Work out the finished part from the listing and answer in its coordinate system (mm). Face numbers are marked on the shaded views. A direction names the side the tool comes from. Give positions to 0.01 mm unless a question says otherwise; leave off trailing zeros. Loops run counter-clockwise (first coordinate to the right, second up) from the corner with the lowest first, then second, coordinate; pieces in that order, holes last. Notation, with made-up numbers: (45.5, 80) - (79.5, 80) arc R23 cw to (79.5, 98) - close; hole circle Ø5 at (45.5, 5.25). An arc over 180 degrees is marked (long way). One line per question, with ' | ' between items.
from build123d import *

# Parameters (mm, degrees)
CUT_CENTER_DEPTH               = 53.414934066
CUT_CENTER_DEPTH_BACK          = 53.414934066
SKETCH_CENTER_CUT_R            = 12.5
CBORE_FOR_M6_SHCS1_D           = 6.6
CBORE_FOR_M6_SHCS1_CBORE_D     = 11
CBORE_FOR_M6_SHCS1_CBORE_DEPTH = 6
CIRPATTERN1_COUNT              = 6
SKETCH1_R                      = 14.25575
CUT_EXTRUDE1_DEPTH             = 3.9624
CUT_EXTRUDE2_DEPTH             = 6
CIRPATTERN2_COUNT              = 6


with BuildPart() as part:
    # Sketch Spindle Skeleton → Main Revolve (revolve)
    with BuildSketch(Plane(origin=(0, 0, 0), x_dir=(0, 0, -1), z_dir=(1, 0, 0)), mode=Mode.PRIVATE) as main_revolve_sk:
        Polygon((-26.320999936, -22.6187), (-26.320999936, -36.5125), (-17.320999902, -36.5125), (-17.320999902, -9.525), (-26.320999936, -9.525), (-26.320999936, -12.5), (-28.321, -12.5), (-28.321, -22.6187), align=None)
        Polygon((-26.320999936, 36.5125), (-26.320999936, 22.6187), (-28.321, 22.6187), (-28.321, 12.5), (-26.320999936, 12.5), (-26.320999936, 9.525), (-17.320999902, 9.525), (-17.320999902, 36.5125), align=None)
    revolve(main_revolve_sk.sketch.rotate(Axis((0, 0, 1000), (0, 0, -1)), 270), axis=Axis((0, 0, 1000), (0, 0, -1)))

    # Sketch Center Cut → Cut Center (cut, two sides: drawn at the far end of the back side and taken through both)
    with BuildSketch(Plane.XY.offset(26.320999936).offset(-CUT_CENTER_DEPTH_BACK)):
        Circle(SKETCH_CENTER_CUT_R)
    extrude(amount=CUT_CENTER_DEPTH + CUT_CENTER_DEPTH_BACK, mode=Mode.SUBTRACT)

    # CBORE for M6 SHCS1 (through all)
    with Locations(Plane(origin=(0, 0, 17.320999902), x_dir=(-1, 0, 0), z_dir=(0, 0, -1))):
        with Locations((0, 30.565600032)):
            cbore_for_m6_shcs1 = CounterBoreHole(CBORE_FOR_M6_SHCS1_D / 2, CBORE_FOR_M6_SHCS1_CBORE_D / 2, CBORE_FOR_M6_SHCS1_CBORE_DEPTH)

    # CirPattern1: CBORE for M6 SHCS1 ×6 about axis
    cirpattern1_axis = Axis((0, 0, 0), (0, 0, 1))
    for i in range(1, CIRPATTERN1_COUNT):
        add(cbore_for_m6_shcs1.rotate(cirpattern1_axis, i * 360 / CIRPATTERN1_COUNT), mode=Mode.SUBTRACT)

    # Sketch1 → Cut-Extrude1 (cut)
    with BuildSketch(Plane(origin=(0, 0, 17.320999902), x_dir=(-1, 0, 0), z_dir=(0, 0, -1))):
        Circle(SKETCH1_R)
    extrude(amount=-CUT_EXTRUDE1_DEPTH, mode=Mode.SUBTRACT)

    # Sketch2 → Cut-Extrude2 (cut)
    with BuildSketch(Plane(origin=(0, 0, 17.320999902), x_dir=(-1, 0, 0), z_dir=(0, 0, -1))):
        with BuildLine():
            ThreePointArc((5.5, 30.565600032), (5.416442642, 29.610535055), (5.168309414, 28.684489244))
            Line((5.168309414, 28.684489244), (7.71724355, 35.687628224))
            ThreePointArc((7.71724355, 35.687628224), (3.88060116, 36.305696397), (0, 36.5125))
            Line((0, 36.5125), (0, 36.065600032))
            ThreePointArc((0, 36.065600032), (3.889087297, 34.454687329), (5.5, 30.565600032))
        make_face()
        with BuildLine():
            Line((-7.71724355, 35.687628224), (-5.168309414, 28.684489244))
            ThreePointArc((-5.168309414, 28.684489244), (-4.505336244, 33.720270432), (0, 36.065600032))
            Line((0, 36.065600032), (0, 36.5125))
            ThreePointArc((0, 36.5125), (-3.88060116, 36.305696397), (-7.71724355, 35.687628224))
        make_face()
    cut_extrude2 = extrude(amount=-CUT_EXTRUDE2_DEPTH, mode=Mode.SUBTRACT)

    # CirPattern2: Cut-Extrude2 ×6 about axis
    cirpattern2_axis = Axis((0, 0, 0), (0, 0, 1))
    for i in range(1, CIRPATTERN2_COUNT):
        add(cut_extrude2.rotate(cirpattern2_axis, i * 360 / CIRPATTERN2_COUNT), mode=Mode.SUBTRACT)


solid = part.part
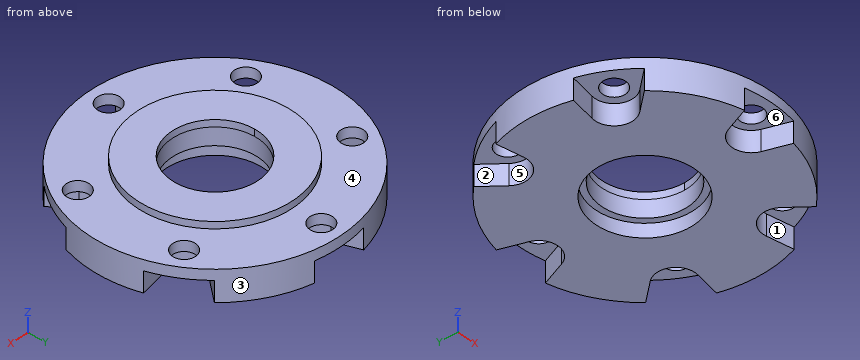
1. Find section A-A on x = 0. Write down the section's boundary in (y, z).
Evaluation:
outline: (-36.51, 23.32) - (-33.87, 23.32) - (-33.87, 26.32) - (-36.51, 26.32) - close; (-27.27, 23.32) - (-25.07, 23.32) - (-25.07, 17.32) - (-14.26, 17.32) - (-14.26, 21.28) - (-12.5, 21.28) - (-12.5, 28.32) - (-22.62, 28.32) - (-22.62, 26.32) - (-27.27, 26.32) - close; (12.5, 21.28) - (14.26, 21.28) - (14.26, 17.32) - (25.07, 17.32) - (25.07, 23.32) - (27.27, 23.32) - (27.27, 26.32) - (22.62, 26.32) - (22.62, 28.32) - (12.5, 28.32) - close; (33.87, 23.32) - (36.51, 23.32) - (36.51, 26.32) - (33.87, 26.32) - close
2. Flat-ended cylindrical pins translate along their axes: pin 1 (4 mm diameter, centred on x = 26.47, y = -15.28, fed in from +Z); pin 2 (1 mm diameter, centred on x = -2, z = 24, fed in from +Y); pin 3 (10.5 mm diameter, centred on x = 0, y = -30.57, fed in from +Z); pin 4 (8.5 mm diameter, centred on x = 0, y = 30.57, fed in from -Z). Find the tip coordinate at first contact, or state that the pin passes through.
Evaluation:
pin 1: through | pin 2: y = 36.48 | pin 3: z = 26.32 | pin 4: z = 23.32
3. Which of the six approach directions +Z, -Z, +X, -X, +Y, -Y give full straight-line access (tool end or side, diameter ignored) to the marked faces 4, 5 and 6?
Evaluation:
face 4: +Z | face 5: -Z | face 6: -Z, -Y
4. Consider L1, parallel to Y at x = 0, z = 24.7; L2, parallel to Y at x = 22.5, z = 18; L3, parallel to Z at x = -16, y = -25. Determine where each line is inside the solid, lowest interval first.
Evaluation:
L1: -36.51 to -33.87, -27.27 to -12.5, 12.5 to 27.27, 33.87 to 36.51 | L2: -28.76 to -19.11, -11.48 to 11.48, 19.11 to 28.76 | L3: 17.32 to 26.32
5. Determine the mould class of the marked faces 1, 2 and 3 for opening direction X: +X half, -X half, draft (parallel to the pull), parting line (faces both ways), or undercut.
Evaluation:
face 1: undercut | face 2: -X half | face 3: parting line
6. Find section B-B on x = -9. Write down the section's boundary in (y, z).
Evaluation:
outline: (-35.39, 17.32) - (-11.06, 17.32) - (-11.06, 21.28) - (-8.67, 21.28) - (-8.67, 28.32) - (-20.75, 28.32) - (-20.75, 26.32) - (-35.39, 26.32) - close; (8.67, 21.28) - (11.06, 21.28) - (11.06, 17.32) - (35.39, 17.32) - (35.39, 26.32) - (20.75, 26.32) - (20.75, 28.32) - (8.67, 28.32) - close
7. Find section C-C on z = 24.5. Write down the section's boundary in (x, y) (1 decimal).
Evaluation:
outline: circle Ø73 at (0, 0); hole circle Ø6.6 at (-26.5, -15.3); hole circle Ø6.6 at (-26.5, 15.3); hole circle Ø25 at (0, 0); hole circle Ø6.6 at (0, -30.6); hole circle Ø6.6 at (0, 30.6); hole circle Ø6.6 at (26.5, -15.3); hole circle Ø6.6 at (26.5, 15.3)
